from build123d import *

# Parameters (mm, degrees)
SKETCH1_W                      = 53.2
SKETCH1_H                      = 26.6
BOSS_EXTRUDE1_DEPTH            = 9.5
SKETCH2_W                      = 50
SKETCH2_H                      = 25
CUT_EXTRUDE1_DEPTH             = 10.5
SKETCH3_W                      = 44
SKETCH3_H                      = 1.6
BOSS_EXTRUDE2_DEPTH            = 50.5
SKETCH4_W                      = 9.5
SKETCH4_H                      = 1.6
BOSS_EXTRUDE3_DEPTH            = 4.6
SKETCH5_W                      = 9.5
SKETCH5_H                      = 1.6
BOSS_EXTRUDE4_DEPTH            = 25
SKETCH6_W                      = 9.5
SKETCH6_H                      = 1.6
BOSS_EXTRUDE5_DEPTH            = 4.6
SKETCH7_W                      = 9.5
SKETCH7_H                      = 1.6
BOSS_EXTRUDE6_DEPTH            = 25
SKETCH8_W                      = 35
SKETCH8_H                      = 1.6
BOSS_EXTRUDE7_DEPTH            = 8
SKETCH9_W                      = 35
SKETCH9_H                      = 1.6
BOSS_EXTRUDE8_DEPTH            = 8
F_8_0_8_DIAMETER_HOLE1_D       = 8
F_8_0_8_DIAMETER_HOLE1_DEPTH   = 26.6
F_3_7_3_7_DIAMETER_HOLE1_D     = 3.7
F_3_7_3_7_DIAMETER_HOLE1_DEPTH = 26.6
F_3_7_3_7_DIAMETER_HOLE2_D     = 3.7
F_3_7_3_7_DIAMETER_HOLE2_DEPTH = 1.6
F_3_7_3_7_DIAMETER_HOLE3_D     = 3.7
F_3_7_3_7_DIAMETER_HOLE3_DEPTH = 56.6
FILLET1_R                      = 0.4
FILLET2_R                      = 2


with BuildPart() as part:
    # Sketch1 → Boss-Extrude1 (new body)
    with BuildSketch(Plane(origin=(60, 0, 0), x_dir=(0, 0, -1), z_dir=(1, 0, 0))):
        with Locations((26.6, 13.3)):
            Rectangle(SKETCH1_W, SKETCH1_H)
    extrude(amount=-BOSS_EXTRUDE1_DEPTH)

    # Sketch2 → Cut-Extrude1 (cut, through all)
    with BuildSketch(Plane.ZY.offset(-50.5)):
        with Locations((-26.6, 14.1)):
            Rectangle(SKETCH2_W, SKETCH2_H)
    extrude(amount=-CUT_EXTRUDE1_DEPTH, mode=Mode.SUBTRACT)

    # Sketch3 → Boss-Extrude2 (add)
    with BuildSketch(Plane.ZY.offset(-50.5)):
        with Locations((-26.6, 0.8)):
            Rectangle(SKETCH3_W, SKETCH3_H)
    extrude(amount=BOSS_EXTRUDE2_DEPTH)

    # Sketch4 → Boss-Extrude3 (add)
    with BuildSketch(Plane(origin=(0, 0, -48.6), x_dir=(-1, 0, 0), z_dir=(0, 0, -1))):
        with Locations((-4.75, 0.8)):
            Rectangle(SKETCH4_W, SKETCH4_H)
    extrude(amount=BOSS_EXTRUDE3_DEPTH)

    # Sketch5 → Boss-Extrude4 (add)
    with BuildSketch(Plane(origin=(0, 1.6, 0), x_dir=(-1, 0, 0), z_dir=(0, 1, 0))):
        with Locations((-4.75, -52.4)):
            Rectangle(SKETCH5_W, SKETCH5_H)
    extrude(amount=BOSS_EXTRUDE4_DEPTH)

    # Sketch6 → Boss-Extrude5 (add)
    with BuildSketch(Plane.XY.offset(-4.6)):
        with Locations((4.75, 0.8)):
            Rectangle(SKETCH6_W, SKETCH6_H)
    extrude(amount=BOSS_EXTRUDE5_DEPTH)

    # Sketch7 → Boss-Extrude6 (add)
    with BuildSketch(Plane(origin=(0, 1.6, 0), x_dir=(-1, 0, 0), z_dir=(0, 1, 0))):
        with Locations((-4.75, -0.8)):
            Rectangle(SKETCH7_W, SKETCH7_H)
    extrude(amount=BOSS_EXTRUDE6_DEPTH)

    # Sketch8 → Boss-Extrude7 (add)
    with BuildSketch(Plane(origin=(0, 0, -48.6), x_dir=(-1, 0, 0), z_dir=(0, 0, -1))):
        with Locations((-30, 0.8)):
            Rectangle(SKETCH8_W, SKETCH8_H)
    extrude(amount=BOSS_EXTRUDE7_DEPTH)

    # Sketch9 → Boss-Extrude8 (add)
    with BuildSketch(Plane.XY.offset(-4.6)):
        with Locations((30, 0.8)):
            Rectangle(SKETCH9_W, SKETCH9_H)
    extrude(amount=BOSS_EXTRUDE8_DEPTH)

    # Ø8.0 (8) Diameter Hole1
    with Locations(Plane(origin=(0, 0, 0), x_dir=(-1, 0, 0), z_dir=(0, -1, 0))):
        with Locations((-22, 42.6), (-22, 10.6), (-38, 42.6), (-38, 10.6)):
            Hole(F_8_0_8_DIAMETER_HOLE1_D / 2, depth=F_8_0_8_DIAMETER_HOLE1_DEPTH)

    # Ø3.7 (3.7) Diameter Hole1
    with Locations(Plane(origin=(0, 0, 0), x_dir=(-1, 0, 0), z_dir=(0, -1, 0))):
        with Locations((-30, 42.6), (-22, 18.6), (-14, 10.6), (-22, 2.6), (-22, 50.6), (-14, 42.6), (-22, 34.6), (-38, 18.6), (-46, 10.6), (-38, 2.6), (-38, 50.6), (-46, 42.6), (-38, 34.6), (-30, 10.6)):
            Hole(F_3_7_3_7_DIAMETER_HOLE1_D / 2, depth=F_3_7_3_7_DIAMETER_HOLE1_DEPTH)

    # Ø3.7 (3.7) Diameter Hole2
    with Locations(Plane(origin=(0, 0, -53.2), x_dir=(-1, 0, 0), z_dir=(0, 0, -1))):
        with Locations((-53.75, 11.6), (-53.75, 21.6), (-6.25, 11.6), (-6.25, 21.6)):
            Hole(F_3_7_3_7_DIAMETER_HOLE2_D / 2, depth=F_3_7_3_7_DIAMETER_HOLE2_DEPTH)

    # Ø3.7 (3.7) Diameter Hole3
    with Locations(Plane.XY):
        with Locations((53.75, 11.6), (53.75, 21.6), (6.25, 11.6), (6.25, 21.6)):
            Hole(F_3_7_3_7_DIAMETER_HOLE3_D / 2, depth=F_3_7_3_7_DIAMETER_HOLE3_DEPTH)

    # Fillet1
    fillet1_edges = [part.edges().sort_by_distance(p)[0] for p in [
        (4.75, 1.6, -51.6),
        (55.25, 1.6, -1.6),
        (4.75, 1.6, -1.6),
        (55.25, 1.6, -51.6),
    ]]
    fillet(fillet1_edges, radius=FILLET1_R)

    # Fillet2
    fillet2_edges = [part.edges().sort_by_distance(p)[0] for p in [
        (4.75, 0, 0),
        (4.75, 0, -53.2),
        (55.25, 0, -53.2),
        (47.5, 0.8, 3.4),
        (60, 26.6, -0.8),
        (12.5, 0.8, -56.6),
        (50.5, 26.6, -52.4),
        (12.5, 0.8, 3.4),
        (60, 26.6, -52.4),
        (55.25, 0, 0),
        (0, 26.6, -52.4),
        (47.5, 0.8, -56.6),
        (9.5, 26.6, -52.4),
        (9.5, 26.6, -0.8),
        (0, 26.6, -0.8),
        (50.5, 26.6, -0.8),
    ]]
    fillet(fillet2_edges, radius=FILLET2_R)


solid = part.part
Design review of the part built by this model. Coordinates are the model's own, in mm. A direction names the side the tool comes from. Round coordinates to 2 decimals unless told otherwise and drop trailing zeros. Loops run counter-clockwise (first coordinate to the right, second up) from the corner with the lowest first, then second, coordinate; pieces in that order, holes last. Notation, with made-up numbers: (74, 42.5) - (104, 42.5) arc R28 cw to (104, 62.5) - close; hole circle Ø8 at (36.5, 52). An arc over 180 degrees is marked (long way). One line per question, with ' | ' between items.
1. Draft analysis for pull direction X (two halves, no side actions). For faces 4 (the face through (0.6, 26.03, -0.79)), 5 (the face through (52.386, 12.85, -52.389)), 6 (the face through (60, 1, -26)), 7 (the face through (5, 14, -53.2)), state which applies: released by +X, released by -X, zero draft, split by the parting line, or undercut.
Results are:
face 4: released by -X | face 5: undercut | face 6: released by +X | face 7: zero draft
2. Clearance check with flat-ended pins moving along their axes: P1, Ø4.5, axis at x = 38, z = -34.6, coming from the +Y side; P2, Ø1.8, axis at x = 49.5, y = 1, coming from the -Z side; P3, Ø4.5, axis at x = 6.25, y = 21.6, coming from the -Z side. State where each tip first meets the part, or that it passes through.
Results are:
P1: stops at y = 1.6 | P2: stops at z = -48.6 | P3: stops at z = -53.2
3. We need section B-B, the plane y = 5.25. State the section outline as (x, z) points.
Results are:
outline: (0, -53.2) - (9.5, -53.2) - (9.5, -51.6) - (0, -51.6) - close; (0, -1.6) - (9.5, -1.6) - (9.5, 0) - (0, 0) - close; (50.5, -53.2) - (60, -53.2) - (60, -51.6) - (50.5, -51.6) - close; (50.5, -1.6) - (60, -1.6) - (60, 0) - (50.5, 0) - close
4. For faces 1 (the face through (49, 1, -48.6)), 2 (the face through (5, 14, -51.6)), 3 (the face through (12.5, 1, -2)), list the 3-axis set-ups (+Z, -Z, +X, -X, +Y, -Y) from which the entire face can be reached by the end or side of a thin tool; tool diameter is ignored.
Results are:
face 1: -Z, +Y, -Y | face 2: +X, -X, +Y | face 3: +Z, +Y, -Y
5. For L1, parallel to X at y = 1.1, z = -18.6; L2, parallel to X at y = 21.6, z = -52.45; L3, parallel to X at y = 0.7, z = -42.6, list the stretches that pass through material, from the lowest coordinate up. Write a range as [from, to].
Results are:
L1: x = [0, 20.15], [23.85, 36.15], [39.85, 60] | L2: x = [0, 4.4], [8.1, 9.5], [50.5, 51.9], [55.6, 60] | L3: x = [0, 12.15], [15.85, 18], [26, 28.15], [31.85, 34], [42, 44.15], [47.85, 60]
6. We need section A-A, the plane z = -42.6. State the section outline as (x, y) points.
Results are:
outline: (0, 0) - (12.15, 0) - (12.15, 1.6) - (0, 1.6) - close; (15.85, 0) - (18, 0) - (18, 1.6) - (15.85, 1.6) - close; (26, 0) - (28.15, 0) - (28.15, 1.6) - (26, 1.6) - close; (31.85, 0) - (34, 0) - (34, 1.6) - (31.85, 1.6) - close; (42, 0) - (44.15, 0) - (44.15, 1.6) - (42, 1.6) - close; (47.85, 0) - (60, 0) - (60, 1.6) - (47.85, 1.6) - close
7. We need section D-D, the plane x = 22. State the section outline as (y, z) points.
Results are:
outline: (0, -56.6) - (1.6, -56.6) - (1.6, -52.45) - (0, -52.45) - close; (0, -48.75) - (1.6, -48.75) - (1.6, -46.6) - (0, -46.6) - close; (0, -38.6) - (1.6, -38.6) - (1.6, -36.45) - (0, -36.45) - close; (0, -32.75) - (1.6, -32.75) - (1.6, -20.45) - (0, -20.45) - close; (0, -16.75) - (1.6, -16.75) - (1.6, -14.6) - (0, -14.6) - close; (0, -6.6) - (1.6, -6.6) - (1.6, -4.45) - (0, -4.45) - close; (0, -0.75) - (1.6, -0.75) - (1.6, 3.4) - (0, 3.4) - close
8. We need section C-C, the plane z = -18.6. State the section outline as (x, y) points, and give its area (3 significant figures).
Results are:
outline: (0, 0) - (20.15, 0) - (20.15, 1.6) - (0, 1.6) - close; (23.85, 0) - (36.15, 0) - (36.15, 1.6) - (23.85, 1.6) - close; (39.85, 0) - (60, 0) - (60, 1.6) - (39.85, 1.6) - close | area: 84.2 mm²
